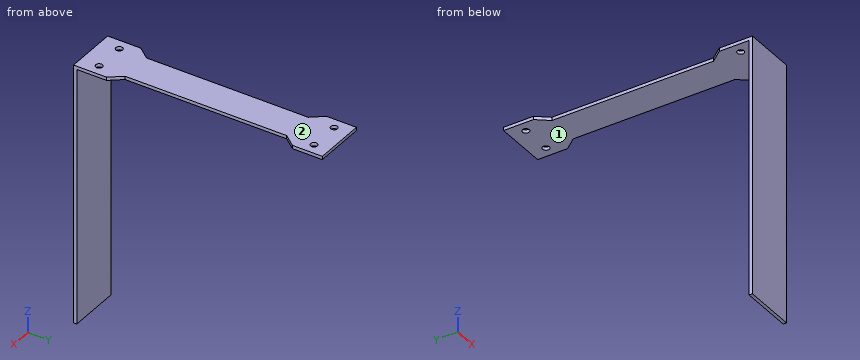
```python
from build123d import *

# Parameters (mm, degrees)
BOSS_EXTRUDE1_DEPTH = 1.5875
SKETCH2_W           = 25.4
SKETCH2_H           = 127
BOSS_EXTRUDE2_DEPTH = 1.5875


with BuildPart() as part:
    # Sketch1 → Boss-Extrude1 (new body)
    with BuildSketch(Plane.XY):
        Polygon((-117, 20.5), (-117, 99.5), (-112.3, 105.418518519), (-112.3, 120), (-137.7, 120), (-137.7, 105.418518519), (-133, 99.5), (-133, 20.5), (-137.7, 14.581481481), (-137.7, 0), (-112.3, 0), (-112.3, 14.581481481), align=None)
        with BuildLine():
            ThreePointArc((-130.85, 7.5), (-132.5, 5.85), (-134.15, 7.5))
            ThreePointArc((-134.15, 7.5), (-132.5, 9.15), (-130.85, 7.5))
        make_face(mode=Mode.SUBTRACT)
        with BuildLine():
            ThreePointArc((-119.15, 7.5), (-117.5, 9.15), (-115.85, 7.5))
            ThreePointArc((-115.85, 7.5), (-117.5, 5.85), (-119.15, 7.5))
        make_face(mode=Mode.SUBTRACT)
        with BuildLine():
            ThreePointArc((-130.85, 112.5), (-132.5, 110.85), (-134.15, 112.5))
            ThreePointArc((-134.15, 112.5), (-132.5, 114.15), (-130.85, 112.5))
        make_face(mode=Mode.SUBTRACT)
        with BuildLine():
            ThreePointArc((-115.85, 112.5), (-117.5, 110.85), (-119.15, 112.5))
            ThreePointArc((-119.15, 112.5), (-117.5, 114.15), (-115.85, 112.5))
        make_face(mode=Mode.SUBTRACT)
    extrude(amount=BOSS_EXTRUDE1_DEPTH)

    # Sketch2 → Boss-Extrude2 (add)
    with BuildSketch(Plane(origin=(0, 0, 0), x_dir=(1, 0, 0), z_dir=(0, 1, 0))):
        with Locations((-125, 61.9125)):
            Rectangle(SKETCH2_W, SKETCH2_H)
    extrude(amount=-BOSS_EXTRUDE2_DEPTH)


solid = part.part
```
Build history of the part. All positions in model axes, mm. Face numbers are marked on the shaded views. A direction names the side the tool comes from. Round coordinates to 2 decimals unless told otherwise and drop trailing zeros. Write each loop counter-clockwise with the first axis right and the second up, starting at its lowest first coordinate (ties: lowest second). Pieces come first, ordered by that corner, then holes. Notation, with made-up numbers: (-18.5, 81.25) - (7.5, 81.25) arc R22 cw to (7.5, 106.25) - close; hole circle Ø10 at (-26, 22.5). An arc over 180 degrees is marked (long way). Answer as CSV lines item,"result".
Q1. Tool access for the marked faces 1 and 2: list every direction of +Z, -Z, +X, -X, +Y, -Y with a clear straight run to the whole face (end or side of a thin tool).
Report:
face 1,"-Z, +X, -X, +Y"
face 2,"+Z, +X, -X, +Y, -Y"
Q2. Drop flat-ended pins along their axis: pin 1 (10 mm diameter, centred on x = -130.5, z = -64, fed in from +Y); pin 2 (8 mm diameter, centred on x = -116, y = 57, fed in from -Z); pin 3 (3 mm diameter, centred on x = -117.5, y = 7.5, fed in from +Z); pin 4 (1.7 mm diameter, centred on y = 43.5, z = 1, fed in from +X). Give the stop position or say it passes through.
Report:
pin 1,"stops at y = 0"
pin 2,"stops at z = 0"
pin 3,"passes through"
pin 4,"stops at x = -117"
Q3. Drill centre lines: probe 1 along Y at (x, z) = (-132.5, 0.7); probe 2 along X at (y, z) = (112, 1); probe 3 along Z at (x, y) = (-128.5, 94.5). Where is each one in solid material? Low to high. Write a range as [from, to].
Report:
probe 1,"y = [-1.59, 5.85], [9.15, 110.85], [114.15, 120]"
probe 2,"x = [-137.7, -134.07], [-130.93, -119.07], [-115.93, -112.3]"
probe 3,"z = [0, 1.59]"
Q4. Cut at C-C (z = -80). Write the cut outline in (x, y).
Report:
outline,"(-137.7, -1.59) - (-112.3, -1.59) - (-112.3, 0) - (-137.7, 0) - close"
Q5. Cut at D-D (x = -122.5). Write the cut outline in (y, z).
Report:
outline,"(-1.59, -125.41) - (0, -125.41) - (0, 0) - (120, 0) - (120, 1.59) - (-1.59, 1.59) - close"
Q6. Cut at A-A (y = 112.5). Write the cut outline in (x, z), and give its area (3 significant figures).
Report:
outline,"(-137.7, 0) - (-134.15, 0) - (-134.15, 1.59) - (-137.7, 1.59) - close; (-130.85, 0) - (-119.15, 0) - (-119.15, 1.59) - (-130.85, 1.59) - close; (-115.85, 0) - (-112.3, 0) - (-112.3, 1.59) - (-115.85, 1.59) - close"
area,"29.8 mm^2"
Q7. Cut at B-B (x = -135.75). Write the cut outline in (y, z).
Report:
outline,"(-1.59, -125.41) - (0, -125.41) - (0, 0) - (17.04, 0) - (17.04, 1.59) - (-1.59, 1.59) - close; (102.96, 0) - (120, 0) - (120, 1.59) - (102.96, 1.59) - close"
